Build history of the part. All positions in model axes, mm. A direction names the side the tool comes from. Coordinates: 2 decimals unless noted, no trailing zeros. Order: outer loops, then holes, each group sorted by start corner. A loop starts at its lowest first (then second) coordinate and runs counter-clockwise, first axis right, second up. Notation, with made-up numbers: (-7, 16) -> (32, 16) arc R23 cw to (32, 30) -> close; hole circle Ø5 at (73, 51). An arc over 180 degrees is marked (long way). Write each question's results on one line, items separated by ' | '.
from build123d import *

# Parameters (mm, degrees)
F1_DEPTH        = 50.8
F3_DEPTH        = 12.7
F5_DEPTH        = 11.938
F7_DEPTH        = 76.2
F8_R            = 6.35
F9_DEPTH        = 6.096
F11_D           = 7.9248
F11_CBORE_D     = 12.7
F11_CBORE_DEPTH = 6.096


with BuildPart() as f1:
    # F0 (on Front) → F1 (new body)
    with BuildSketch(Plane.XZ):
        Polygon((0, 12.7), (0, 0), (91.2594877579, 0), (87.5397438789, 3.7197438789), (96.52, 12.7), align=None)
        Polygon((87.5397438789, 3.7197438789), (91.2594877579, 0), (96.52, 0), (96.52, 12.7), align=None)
        Polygon((96.52, 0), (91.2594877579, 0), (128.3101066686, -37.0506189107), (137.2903627897, -28.0703627897), (96.52, 12.7), align=None)
    extrude(amount=F1_DEPTH)

    # F2 (on face) → F3 (join)
    with BuildSketch(Plane(origin=(54.61, 0, 54.61), x_dir=(0.7071067812, 0, -0.7071067812), z_dir=(0.7071067812, 0, 0.7071067812))):
        with BuildLine():
            Line((116.9276903991, 0), (116.9276903991, -50.8))
            ThreePointArc((116.9276903991, -50.8), (123.2946720443, -25.4), (116.9276903991, 0))
        make_face()
    extrude(amount=-F3_DEPTH)

    # F4 (on face) → F5 (join)
    with BuildSketch(Plane(origin=(54.61, 0, 54.61), x_dir=(0.7071067812, 0, -0.7071067812), z_dir=(0.7071067812, 0, 0.7071067812))):
        with BuildLine():
            Line((66.1276903991, -50.8), (116.9276903991, -50.8))
            ThreePointArc((116.9276903991, -50.8), (123.2946720443, -25.4), (116.9276903991, 0))
            Line((116.9276903991, 0), (66.1276903991, 0))
            Line((66.1276903991, 0), (66.1276903991, -50.8))
        make_face()
    extrude(amount=F5_DEPTH)

    # F6 (on face) → F7 (cut)
    with BuildSketch(Plane(origin=(46.7593383054, 0, -46.7593383054), x_dir=(0, -1, 0), z_dir=(-0.7071067812, 0, 0.7071067812))):
        Polygon((35.052, 89.1682026412), (25.4, 89.1682026412), (15.748, 89.1682026412), (15.748, 83.0722026412), (9.652, 83.0722026412), (9.652, 76.4682026412), (41.148, 76.4682026412), (41.148, 83.0722026412), (35.052, 83.0722026412), align=None)
    extrude(amount=-F7_DEPTH, mode=Mode.SUBTRACT)

    # F8 (on face) → F9 (cut)
    with BuildSketch(Plane(origin=(0, 0, 0), x_dir=(1, 0, 0), z_dir=(0, 0, -1))):
        with Locations((15.748, 38.1)):
            Circle(F8_R)
        with Locations((15.748, 12.7030098811)):
            Circle(F8_R)
        with Locations((69.596, 38.1)):
            Circle(F8_R)
        with Locations((69.596, 12.7030098811)):
            Circle(F8_R)
    extrude(amount=-F9_DEPTH, mode=Mode.SUBTRACT)

    # F11 (through all)
    with Locations(Plane(origin=(0, 0, 0), x_dir=(1, 0, 0), z_dir=(0, 0, -1))):
        with Locations((15.748, 38.1), (69.596, 38.1), (69.596, 12.7030098811), (15.748, 12.7030098811)):
            CounterBoreHole(F11_D / 2, F11_CBORE_D / 2, F11_CBORE_DEPTH)


solid = f1.part
Item 1: Drill centre lines: line 1 (Y direction, x = 112, z = 7); line 2 (X direction, y = -38.1, z = 10.25); line 3 (Z direction, x = 36, y = -39). Where is each one in solid material? Low to high. Write a range as from..to.
Answer:
line 1: y = -50.8..-35.05, -15.75..0 | line 2: x = 0..11.79, 19.71..65.63, 73.56..98.97, 107.23..115.85 | line 3: z = 0..12.7
Item 2: Pull direction Y, two halves, no side cores. Call faces 1 (the flat face through (98.91, -25.04, 10.31)), 2 (the flat face through (87, 0, 4)), 3 (the flat face through (122, -9.652, -9)): released by +Y, released by -Y, zero draft, split by the parting line, or undercut.
Answer:
face 1: zero draft | face 2: released by +Y | face 3: undercut
Item 3: Slice it at D-D, the plane z = 2. List the corners of the cut face in (x, y).
Answer:
outline: (0, -50.8) -> (124.1, -50.8) -> (124.1, -35.05) -> (115.48, -35.05) -> (115.48, -41.15) -> (106.14, -41.15) -> (106.14, -9.65) -> (115.48, -9.65) -> (115.48, -15.75) -> (124.1, -15.75) -> (124.1, 0) -> (0, 0) -> close; hole circle Ø12.7 at (15.75, -38.1); hole circle Ø12.7 at (15.75, -12.7); hole circle Ø12.7 at (69.6, -38.1); hole circle Ø12.7 at (69.6, -12.7)
Item 4: Slice it at A-A, the plane y = -38.1. List the corners of the cut face in (x, z), and give its area (3 significant figures).
Answer:
outline: (0, 0) -> (9.4, 0) -> (9.4, 6.1) -> (11.79, 6.1) -> (11.79, 12.7) -> (0, 12.7) -> close; (19.71, 6.1) -> (22.1, 6.1) -> (22.1, 0) -> (63.25, 0) -> (63.25, 6.1) -> (65.63, 6.1) -> (65.63, 12.7) -> (19.71, 12.7) -> close; (73.56, 6.1) -> (75.95, 6.1) -> (75.95, 0) -> (91.26, 0) -> (131.74, -40.48) -> (140.18, -32.04) -> (100.83, 7.31) -> (101.37, 7.85) -> (96.52, 12.7) -> (73.56, 12.7) -> close; (105.5, 11.98) -> (144.85, -27.37) -> (149.16, -23.06) -> (109.81, 16.29) -> close | area: 1,990 mm^2
Item 5: Slice it at B-B, the plane z = -17. List the corners of the cut face in (x, y), and give its area (3 significant figures).
Answer:
outline: (108.26, -50.8) -> (143.1, -50.8) -> (143.1, -35.05) -> (134.48, -35.05) -> (134.48, -41.15) -> (125.14, -41.15) -> (125.14, -9.65) -> (134.48, -9.65) -> (134.48, -15.75) -> (143.1, -15.75) -> (143.1, 0) -> (108.26, 0) -> close | area: 1,310 mm^2
Item 6: Slice it at C-C, the plane y = -29. List the corners of the cut face in (x, z).
Answer:
outline: (0, 0) -> (91.26, 0) -> (132.73, -41.47) -> (141.17, -33.03) -> (100.83, 7.31) -> (101.37, 7.85) -> (96.52, 12.7) -> (0, 12.7) -> close
Item 7: Pin check, flat tips, straight feed: pin 1 (10.5 mm diameter, centred on x = 15.75, y = -12.7, fed in from +Z); pin 2 (10 mm diameter, centred on x = 66, y = -30, fed in from -Z); pin 3 (6.5 mm diameter, centred on x = 70, y = -41, fed in from -Z). Stop position of each tip, or through.
Answer:
pin 1: stops at z = 12.7 | pin 2: stops at z = 0 | pin 3: stops at z = 6.1
Item 8: Tool access for faces 4 (the flat face through (106.47, -44.57, 12.95)), 5 (the flat face through (120.76, -25.18, -12.62)), 6 (the cylindrical face through (21.805, -14.61, 3.005)), 7 (the flat face through (49, -25, 12.7)), 8 (the flat face through (127, -15.748, -5)): list every direction of +Z, -Z, +X, -X, +Y, -Y with a clear straight run to the whole face (end or side of a thin tool).
Answer:
face 4: +Z, +Y, -Y | face 5: none | face 6: -Z | face 7: +Z, -X, +Y, -Y | face 8: +Z, +X
